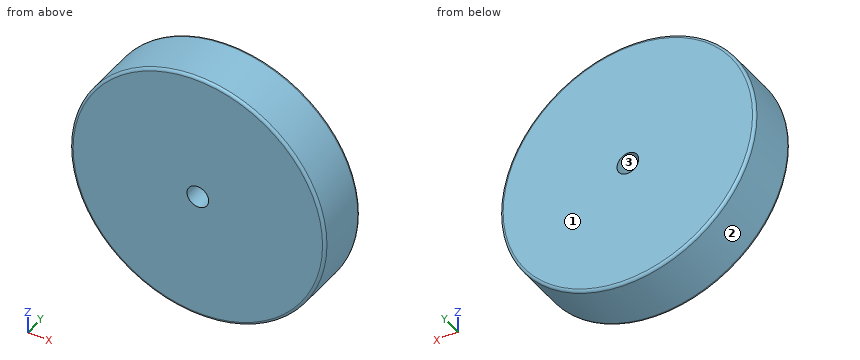
from build123d import *

# Parameters (mm, degrees)
F0_R     = 23.5
F1_DEPTH = 10
F2_R     = 2
F3_DEPTH = 25.4
F4_R     = 0.5


with BuildPart() as f1:
    # F0 (on Front) → F1 (new body)
    with BuildSketch(Plane.XZ):
        Circle(F0_R)
    extrude(amount=F1_DEPTH)

    # F2 (on face) → F3 (cut)
    with BuildSketch(Plane.XZ.offset(10)):
        Circle(F2_R)
    extrude(amount=-F3_DEPTH, mode=Mode.SUBTRACT)

    # F4
    f4_edges = [f1.edges().sort_by_distance(p)[0] for p in [
        (-23.5, -10, 0),
        (-23.5, 0, 0),
    ]]
    fillet(f4_edges, radius=F4_R)


solid = f1.part
The listing builds one solid part. Answer for the finished solid, in the listing's coordinates (mm). Face numbers are marked on the shaded views. Coordinates: 2 decimals unless noted, no trailing zeros. Write each loop counter-clockwise with the first axis right and the second up, starting at its lowest first coordinate (ties: lowest second). Pieces come first, ordered by that corner, then holes. Notation, with made-up numbers: (-9.5, -5) -> (21.5, -5) arc R16 ccw to (21.5, 10) -> close; hole circle Ø10 at (50, 47). An arc over 180 degrees is marked (long way). One line per question, with ' | ' between items.
1. Section C-C (y = -4) is taken. Determine the outline of the cut face in (x, z).
Verdict:
outline: circle Ø47 at (0, 0); hole circle Ø4 at (0, 0)
2. Straight lines are drawn through the part: line 1 (Z direction, x = 0, y = -4.75); line 2 (Z direction, x = 19, y = -2); line 3 (X direction, y = -3.5, z = 15.5). For each, find the intervals that lie inside material, in ascending order.
Verdict:
line 1: z = -23.5 to -2, 2 to 23.5 | line 2: z = -13.83 to 13.83 | line 3: x = -17.66 to 17.66
3. Section B-B (z = 0) is taken. Determine the outline of the cut face in (x, y).
Verdict:
outline: (-23.5, -9.5) arc R0.5 ccw to (-23, -10) -> (-2, -10) -> (-2, 0) -> (-23, 0) arc R0.5 ccw to (-23.5, -0.5) -> close; (2, -10) -> (23, -10) arc R0.5 ccw to (23.5, -9.5) -> (23.5, -0.5) arc R0.5 ccw to (23, 0) -> (2, 0) -> close
4. For a pull along X with two mould halves and no side action, classify the marked faces 1, 2 and 3 as released by +X, released by -X, zero draft, split by the parting line, or undercut.
Verdict:
face 1: zero draft | face 2: split by the parting line | face 3: undercut
5. Given pin 1 Ø4 at (x, y) = (15, -6.5) entering from +Z; pin 2 Ø2.5 at (x, z) = (0, 0) entering from +Y; pin 3 Ø5 at (x, y) = (17.5, -1) entering from +Z; pin 4 Ø1.5 at (x, y) = (-14, -2.5) entering from -Z, each flat-ended and moving along its own axis, determine where each tip first touches the part or whether it passes through.
Verdict:
pin 1: stops at z = 19.58 | pin 2: passes through | pin 3: stops at z = 18.09 | pin 4: stops at z = -19.41
6. Section A-A (x = 0) is taken. Determine the outline of the cut face in (y, z).
Verdict:
outline: (-10, -23) arc R0.5 ccw to (-9.5, -23.5) -> (-0.5, -23.5) arc R0.5 ccw to (0, -23) -> (0, -2) -> (-10, -2) -> close; (-10, 2) -> (0, 2) -> (0, 23) arc R0.5 ccw to (-0.5, 23.5) -> (-9.5, 23.5) arc R0.5 ccw to (-10, 23) -> close
